from build123d import *

# Parameters (mm, degrees)
SKETCH2_R           = 10
BOSS_EXTRUDE1_DEPTH = 1.75
BOSS_EXTRUDE2_DEPTH = 2.5
CUT_EXTRUDE1_START  = -2.5
CUT_EXTRUDE1_DEPTH  = 2.5


with BuildPart() as part:
    # Sketch2 → Boss-Extrude1 (new body)
    with BuildSketch(Plane(origin=(0, 0, 0), x_dir=(1, 0, 0), z_dir=(0, 1, 0))):
        with Locations(Location((0, 0, 0), (0, 0, 270))):
            Circle(SKETCH2_R)
    extrude(amount=BOSS_EXTRUDE1_DEPTH)

    # Sketch3 → Boss-Extrude2 (add)
    with BuildSketch(Plane.XZ):
        with BuildLine():
            Line((-4.25, 0), (-0.138270177, -4.111729823))
            Line((-0.138270177, -4.111729823), (4.119266685, 0.145807039))
            Line((4.119266685, 0.145807039), (0, 4.25))
            ThreePointArc((0, 4.25), (4.25, 0), (0, -4.25))
            ThreePointArc((0, -4.25), (-3.00520382, -3.00520382), (-4.25, 0))
        make_face()
    extrude(amount=BOSS_EXTRUDE2_DEPTH)

    # Sketch4 → Cut-Extrude1 (cut)
    with BuildSketch(Plane.XZ.offset(CUT_EXTRUDE1_START)):
        with BuildLine():
            Line((-0.138270177, -4.111729823), (4.119266685, 0.145807039))
            Line((4.119266685, 0.145807039), (0, 4.25))
            ThreePointArc((0, 4.25), (-3.00520382, 3.00520382), (-4.25, 0))
            Line((-4.25, 0), (-0.138270177, -4.111729823))
        make_face()
    extrude(amount=CUT_EXTRUDE1_DEPTH, mode=Mode.SUBTRACT)


solid = part.part
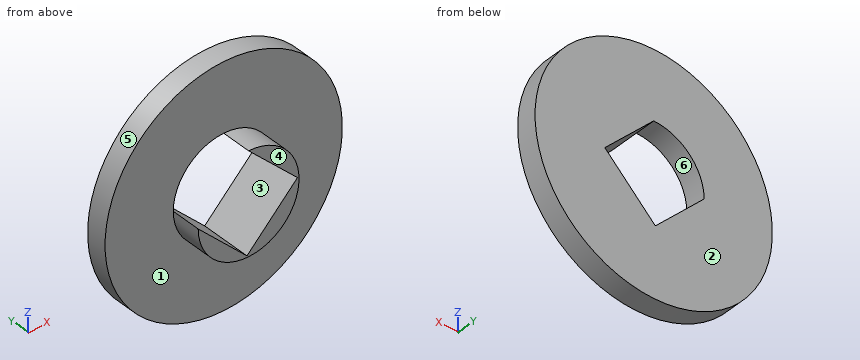
Design review of the part built by this model. Coordinates are the model's own, in mm. Face numbers are marked on the shaded views. A direction names the side the tool comes from. Coordinates: 2 decimals unless noted, no trailing zeros. Order: outer loops, then holes, each group sorted by start corner. A loop starts at its lowest first (then second) coordinate and runs counter-clockwise, first axis right, second up. Notation, with made-up numbers: (18, -26.5) -> (54, -26.5) arc R18 ccw to (54, 7.5) -> close; hole circle Ø1 at (72.5, 76). An arc over 180 degrees is marked (long way). One line per item, written item: value.
1) We need section B-B, the plane x = -4. Give the boundary of the cut face in (y, z), then the cut area to 3 significant figures.
Output values:
outline: (-2.5, -1.44) -> (0, -1.44) -> (0, -9.17) -> (1.75, -9.17) -> (1.75, -0.25) -> (-2.5, -0.25) -> close; (0, 1.44) -> (1.75, 1.44) -> (1.75, 9.17) -> (0, 9.17) -> close
area: 32.1 mm2
2) Machinability: for the marked faces 1 and 2, which of the approach directions +Z, -Z, +X, -X, +Y, -Y give a long, thin tool a straight path to every point of the face, cutting with its end or side? Answer none if there is none.
Output values:
face 1: -Y
face 2: +Z, -Z, +X, -X, +Y
3) We need section C-C, the plane y = -1.1. Give the boundary of the cut face in (x, z), then the cut area to 3 significant figures.
Output values:
outline: (-4.25, 0) arc R4.25 ccw (long way) to (0, 4.25) -> (4.12, 0.15) -> (-0.14, -4.11) -> close
area: 16.6 mm2
4) To check wall thickness, follow probe 1 along Y at (x, z) = (5, 8); probe 2 along X at (y, z) = (1.35, 0.5); probe 3 along Z at (x, y) = (1, -1.5). State the ranges of each line that lie inside material, in increasing order. Write a range as [from, to].
Output values:
probe 1: y = [0, 1.75]
probe 2: x = [-9.99, -4.22], [3.76, 9.99]
probe 3: z = [-4.13, -2.97], [3.25, 4.13]
5) We need section A-A, the plane z = -1.25. Give the boundary of the cut face in (x, y).
Output values:
outline: (-9.92, 0) -> (-4.06, 0) -> (-4.06, -2.5) -> (-3, -2.5) -> (-3, 1.75) -> (-9.92, 1.75) -> close; (2.72, -2.5) -> (4.06, -2.5) -> (4.06, 0) -> (9.92, 0) -> (9.92, 1.75) -> (2.72, 1.75) -> close
6) Draft analysis for pull direction Z (two halves, no side actions). For the marked faces 3, 4, 5 and 6, state which applies: +Z half, -Z half, draft (parallel to the pull), parting line (faces both ways), or undercut.
Output values:
face 3: undercut
face 4: draft
face 5: parting line
face 6: undercut
7) Clearance check with flat-ended pins moving along their axes: P1, Ø2, axis at x = -3, y = 0.5, coming from the -Z side; P2, Ø1, axis at x = -5, y = 1.5, coming from the +Z side. State where each tip first meets the part, or that it passes through.
Output values:
P1: stops at z = -9.8
P2: stops at z = 8.93
8) We need section D-D, the plane z = 4.5. Give the boundary of the cut face in (x, y), then the cut area to 3 significant figures.
Output values:
outline: (-8.93, 0) -> (8.93, 0) -> (8.93, 1.75) -> (-8.93, 1.75) -> close
area: 31.3 mm2
